Model file for the job. Use its own axes, mm. Face numbers are marked on the shaded views. A direction names the side the tool comes from. Round coordinates to 2 decimals unless told otherwise and drop trailing zeros. Loops run counter-clockwise (first coordinate to the right, second up) from the corner with the lowest first, then second, coordinate; pieces in that order, holes last. Notation, with made-up numbers: M -21,-26 L 22,-26 A18 cw 22,-11 Z; hole C 27.25,0.25 d10. An arc over 180 degrees is marked long. Use a Markdown table: item, result. Add a question column.
Item 1: Saw through at C-C on x = -8.25. Write the cut outline in (y, z).
Item 2: Two-plate mould, pull along Z, no slides. Class the marked faces 4, 5, 6 and 7: +Z half, -Z half, draft (parallel to the pull), parting line (faces both ways), or undercut.
Item 3: Saw through at B-B on y = 1. Write the cut outline in (x, z).
Item 4: Saw through at A-A on x = -10.5. Write the cut outline in (y, z), then the cut area to 3 significant figures.
Item 5: Tool access for the marked faces 1, 2 and 3: list every direction of +Z, -Z, +X, -X, +Y, -Y with a clear straight run to the whole face (end or side of a thin tool).
Item 6: Wall check: L1, parallel to Z at x = -9.75, y = -4; L2, parallel to Z at x = -10, y = -1.25; L3, parallel to Y at x = -7, z = -0.25. Give the ranges that are in metal, low to high. Write a range as from..to.
Item 7: Saw through at D-D on y = -4. Write the cut outline in (x, z).
Item 8: Pin check, flat tips, straight feed: P1, Ø4, axis at y = -2, z = 7.5, coming from the +X side; P2, Ø6, axis at x = -11, z = -1.5, coming from the +Y side. Stop position of each tip, or through.
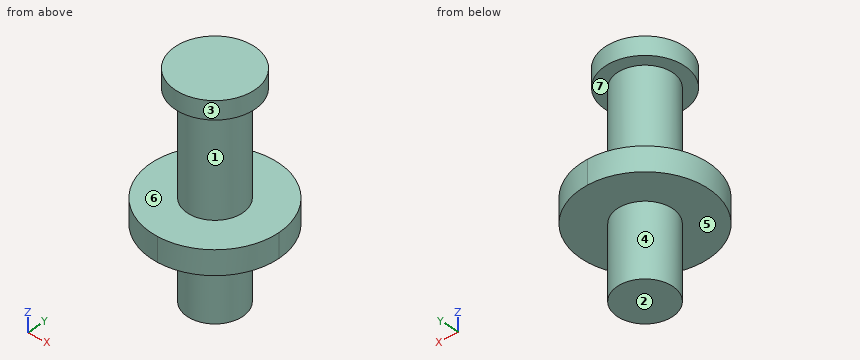
```python
from build123d import *

# Parameters (mm, degrees)
F0_R          = 3.3
F0_R_2        = 2.3
F1_DEPTH      = 2
F2_DEPTH      = 10
F2_DEPTH_BACK = 8
F3_START      = 8.5
F3_DEPTH      = 1.5


with BuildPart() as f1:
    # F0 (on Top) → F1 (new body)
    with BuildSketch(Plane.XY):
        with BuildLine():
            ThreePointArc((-2.2, 0), (-3.7523340597, 3.7476659403), (-7.5, 5.3))
            ThreePointArc((-7.5, 5.3), (-12.8, 0), (-7.5, -5.3))
            ThreePointArc((-7.5, -5.3), (-3.7523340597, -3.7476659403), (-2.2, 0))
        make_face()
        with Locations((-7.5, 0)):
            Circle(F0_R, mode=Mode.SUBTRACT)
        with Locations((-7.5, 0)):
            Circle(F0_R)
        with Locations((-7.5, 0)):
            Circle(F0_R_2, mode=Mode.SUBTRACT)
    extrude(amount=-F1_DEPTH)

    # F0 (on Top) → F2 (join, two sides)
    with BuildSketch(Plane.XY) as f2_sk:
        with Locations((-7.5, 0)):
            Circle(F0_R_2)
    extrude(amount=F2_DEPTH)
    extrude(f2_sk.sketch, amount=-F2_DEPTH_BACK)

    # F0 (on Top) → F3 (join)
    with BuildSketch(Plane.XY.offset(F3_START)):
        with Locations((-7.5, 0)):
            Circle(F0_R)
        with Locations((-7.5, 0)):
            Circle(F0_R_2, mode=Mode.SUBTRACT)
    extrude(amount=F3_DEPTH)


solid = f1.part
```
Entries:
| question | item | result |
|---|---|---|
| 1 | outline | M -5.25,-2 L -2.17,-2 L -2.17,-8 L 2.17,-8 L 2.17,-2 L 5.25,-2 L 5.25,0 L 2.17,0 L 2.17,8.5 L 3.21,8.5 L 3.21,10 L -3.21,10 L -3.21,8.5 L -2.17,8.5 L -2.17,0 L -5.25,0 Z |
| 2 | face 4 | draft |
| 2 | face 5 | -Z half |
| 2 | face 6 | undercut |
| 2 | face 7 | undercut |
| 3 | outline | M -12.7,-2 L -9.57,-2 L -9.57,-8 L -5.43,-8 L -5.43,-2 L -2.3,-2 L -2.3,0 L -5.43,0 L -5.43,8.5 L -4.36,8.5 L -4.36,10 L -10.64,10 L -10.64,8.5 L -9.57,8.5 L -9.57,0 L -12.7,0 Z |
| 4 | outline | M -4.37,-2 L 4.37,-2 L 4.37,0 L -4.37,0 Z; M -1.37,8.5 L 1.37,8.5 L 1.37,10 L -1.37,10 Z |
| 4 | area | 21.6 mm2 |
| 5 | face 1 | none |
| 5 | face 2 | -Z, +X, -X, +Y, -Y |
| 5 | face 3 | +Z |
| 6 | L1 | -2..0 |
| 6 | L2 | -2..0, 8.5..10 |
| 6 | L3 | -5.28..5.28 |
| 7 | outline | M -10.98,-2 L -4.02,-2 L -4.02,0 L -10.98,0 Z |
| 8 | P1 | x = -4.21 |
| 8 | P2 | y = 5.28 |
